Design review of the part shown in the three views and the two pictorial views. Dimensions are in mm from the part's minimum x, y and z. A direction names the side the tool comes from. Round coordinates to 2 decimals unless told otherwise and drop trailing zeros. Loops run counter-clockwise (first coordinate to the right, second up) from the corner with the lowest first, then second, coordinate; pieces in that order, holes last. Notation, with made-up numbers: M 20.25,39 L 29.25,39 A16 ccw 29.25,69 Z; hole C 71.25,-31 d5. An arc over 180 degrees is marked long. Return JSON: item names as keys, results as strings. Group by question number.
Q1. For the marked faces 1, 2 and 3, list the 3-axis set-ups (+Z, -Z, +X, -X, +Y, -Y) from which the entire face can be reached by the end or side of a thin tool; tool diameter is ignored.
Q2. Consider section C-C (x = 60). State the section outline as (y, z) points, and give its area (3 significant figures).
Q3. Clearance check with flat-ended pins moving along their axes: pin 1 Ø3 at (y, z) = (20, 52) entering from -X; pin 2 Ø1.5 at (y, z) = (29, 41.5) entering from +X (3 decimals). State where each tip first meets the part, or that it passes through.
Q4. Consider section D-D (y = 28.5). State the section outline as (x, z) points.
Q5. Consider section B-B (z = 38). State the section outline as (x, y) points, and give its area (3 significant figures).
Q6. Draft analysis for pull direction X (two halves, no side actions). For the marked faces 4, 5 and 6, state which applies: pulls with the +X half, pulls with the -X half, needs draft (parallel to the pull), parting line crosses it, or undercut.
Q7. To check wall thickness, follow line 1 along X through (y, z) = (9.5, 19.5); line 2 along Y through (x, z) = (17.5, 33); line 3 along X through (y, z) = (32.5, 34). State the ranges of each line that lie inside material, in increasing order.
Q8. Consider section A-A (y = 7). State the section outline as (x, z) points, and give its area (3 significant figures).
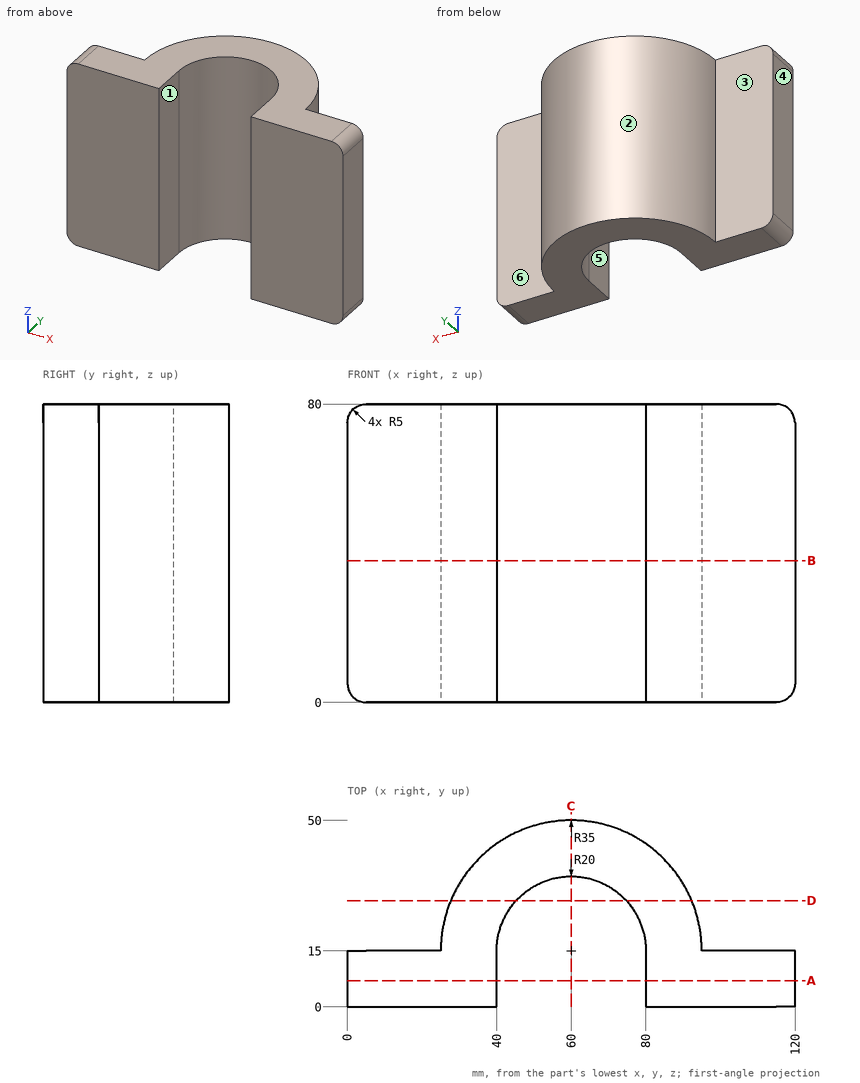
Values:
{
 "1": {"face 1": "+Z, -Z, -Y", "face 2": "+Z, -Z, +Y", "face 3": "+Z, -Z, -X, +Y"},
 "2": {"outline": "M 35,0 L 50,0 L 50,80 L 35,80 Z", "area": "1,200 mm2"},
 "3": {"pin 1": "stops at x = 25.18", "pin 2": "stops at x = 92.395"},
 "4": {"outline": "M 27.71,0 L 45.24,0 L 45.24,80 L 27.71,80 Z; M 74.76,0 L 92.29,0 L 92.29,80 L 74.76,80 Z"},
 "5": {"outline": "M 0,0 L 40,0 L 40,15 A20 cw 80,15 L 80,0 L 120,0 L 120,15 L 95,15 A35 ccw 25,15 L 0,15 Z", "area": "2,500 mm2"},
 "6": {"face 4": "pulls with the -X half", "face 5": "undercut", "face 6": "needs draft"},
 "7": {"line 1": "x = 0 to 40, 80 to 120", "line 2": "y = 0 to 15", "line 3": "x = 29.69 to 50.32, 69.68 to 90.31"},
 "8": {"outline": "M 0,5 A5 ccw 5,0 L 40,0 L 40,80 L 5,80 A5 ccw 0,75 Z; M 80,0 L 115,0 A5 ccw 120,5 L 120,75 A5 ccw 115,80 L 80,80 Z", "area": "6,380 mm2"}
}
